For this review, use the dimensioned drawing (mm, ordinates from the lowest corner) and the shaded views. Give positions to 0.01 mm unless a question says otherwise; leave off trailing zeros. Order: outer loops, then holes, each group sorted by start corner. A loop starts at its lowest first (then second) coordinate and runs counter-clockwise, first axis right, second up. Notation, with made-up numbers: M -19,47.25 L 4,47.25 A11 ccw 4,55.25 Z; hole C 31,68 d5. An arc over 180 degrees is marked long. Use CSV: the item, a comma, the result in double quotes. Start each with the question number.
(1) Wall thickness on L1, parallel to X at y = 5, z = 180; L2, parallel to Z at x = 90, y = 6; L3, parallel to X at y = 7.75, z = 345: over which ranges is each line inside the solid? List them lowest first. Write a range as from..to.
(2) Consider section A-A (x = 90). Write out the cut boundary in (y, z), and give its area (3 significant figures).
(3) Clearance check with a flat-ended pin moving along its axis: P1, Ø6.5, axis at x = 165, z = 345, coming from the +Y side. State where the tip first meets the part, or that it passes through.
(4) Consider section C-C (y = 8). Give the number of separate pieces and of enclosed holes in the cut face, and give its area (3 significant figures).
(5) Consider section B-B (z = 15). Write out the cut boundary in (x, y).
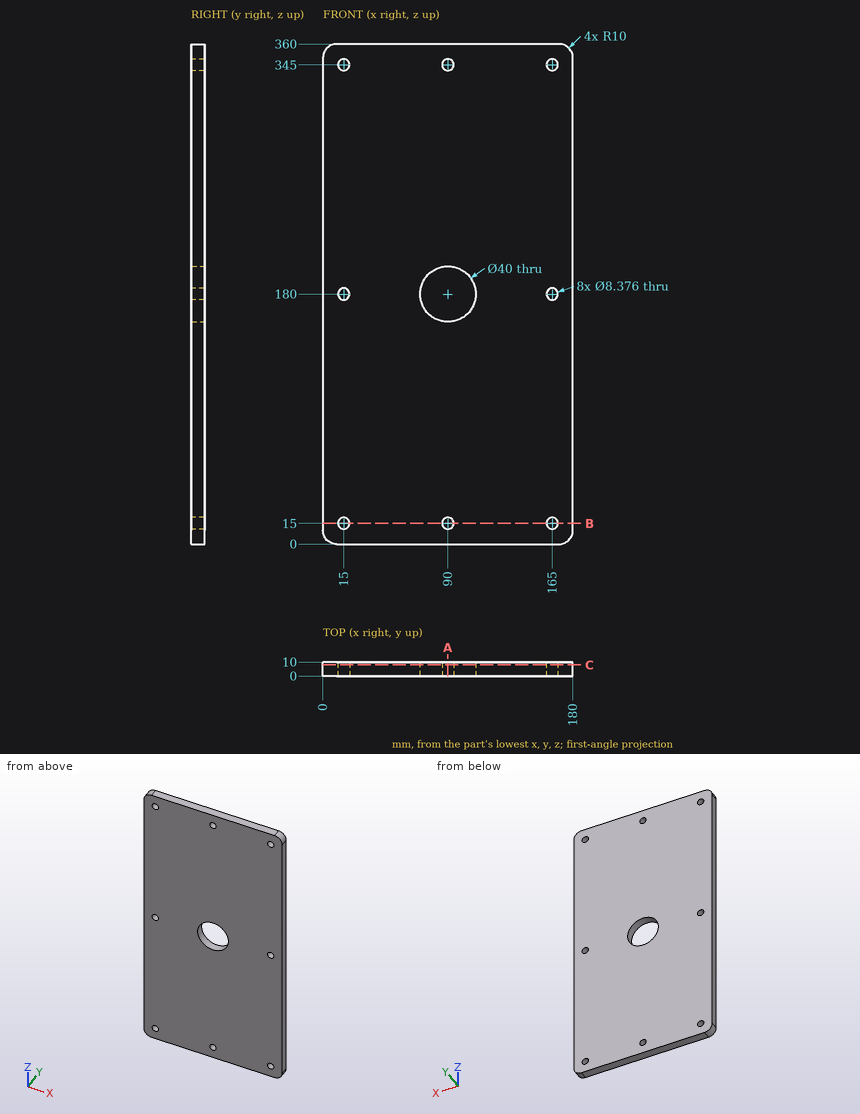
Check result:
1,L1,"x = 0..10.81, 19.19..70, 110..160.81, 169.19..180"
1,L2,"z = 0..10.81, 19.19..160, 200..340.81, 349.19..360"
1,L3,"x = 0..10.81, 19.19..85.81, 94.19..160.81, 169.19..180"
2,outline,"M 0,0 L 10,0 L 10,10.81 L 0,10.81 Z; M 0,19.19 L 10,19.19 L 10,160 L 0,160 Z; M 0,200 L 10,200 L 10,340.81 L 0,340.81 Z; M 0,349.19 L 10,349.19 L 10,360 L 0,360 Z"
2,area,"3,030 mm^2"
3,P1,"passes through"
4,separate pieces,"1"
4,enclosed holes,"9"
4,area,"63,000 mm^2"
5,outline,"M 0,0 L 10.81,0 L 10.81,10 L 0,10 Z; M 19.19,0 L 85.81,0 L 85.81,10 L 19.19,10 Z; M 94.19,0 L 160.81,0 L 160.81,10 L 94.19,10 Z; M 169.19,0 L 180,0 L 180,10 L 169.19,10 Z"
